from build123d import *

# Parameters (mm, degrees)
BOSS_EXTRUDE1_DEPTH     = 202
FILLET1_R               = 1.44
FILLET2_R               = 1.44
SKETCH2_R               = 1.59
SKETCH2_R_2             = 1.735
SKETCH2_R_3             = 1.57
CUT_EXTRUDE1_DEPTH      = 6.1
CUT_EXTRUDE1_DEPTH_BACK = 11.04
FILLET3_R               = 1.44
BOSS_EXTRUDE2_DEPTH     = 202
CUT_EXTRUDE2_DEPTH      = 203
SKETCH5_R               = 1.59
CUT_EXTRUDE3_DEPTH      = 10
SKETCH6_R               = 1.59
BOSS_EXTRUDE3_DEPTH     = 1.59


with BuildPart() as part:
    # Sketch1 → Boss-Extrude1 (new body)
    with BuildSketch(Plane(origin=(0, 0, 0), x_dir=(0, 0, -1), z_dir=(1, 0, 0))):
        with BuildLine():
            Line((-15.04, 0), (15.04, 0))
            Line((15.04, 0), (15.19, 0))
            ThreePointArc((15.19, 0), (16.208233765, 0.421766235), (16.63, 1.44))
            Line((16.63, 1.44), (16.63, 12.11))
            ThreePointArc((16.63, 12.11), (17.051766235, 13.128233765), (18.07, 13.55))
            Line((18.07, 13.55), (24.5, 13.55))
            Line((24.5, 13.55), (24.5, 15.14))
            Line((24.5, 15.14), (16.48, 15.14))
            ThreePointArc((16.48, 15.14), (15.461766235, 14.718233765), (15.04, 13.7))
            Line((15.04, 13.7), (15.04, 3.03))
            ThreePointArc((15.04, 3.03), (14.618233765, 2.011766235), (13.6, 1.59))
            Line((13.6, 1.59), (-13.6, 1.59))
            ThreePointArc((-13.6, 1.59), (-14.618233765, 2.011766235), (-15.04, 3.03))
            Line((-15.04, 3.03), (-15.04, 8.6))
            ThreePointArc((-15.04, 8.6), (-15.461766235, 9.618233765), (-16.48, 10.04))
            Line((-16.48, 10.04), (-24.68, 10.04))
            Line((-24.68, 10.04), (-24.68, 8.45))
            Line((-24.68, 8.45), (-18.07, 8.45))
            ThreePointArc((-18.07, 8.45), (-17.051766235, 8.028233765), (-16.63, 7.01))
            Line((-16.63, 7.01), (-16.63, 1.44))
            ThreePointArc((-16.63, 1.44), (-16.208233765, 0.421766235), (-15.19, 0))
            Line((-15.19, 0), (-15.04, 0))
        make_face()
    extrude(amount=-BOSS_EXTRUDE1_DEPTH)

    # Fillet1
    fillet1_edges = [part.edges().sort_by_distance(p)[0] for p in [
        (0, 9.245, 24.68),
    ]]
    fillet(fillet1_edges, radius=FILLET1_R)

    # Fillet2
    fillet2_edges = [part.edges().sort_by_distance(p)[0] for p in [
        (-202, 14.345, -24.5),
        (0, 14.345, -24.5),
        (-202, 9.245, 24.68),
    ]]
    fillet(fillet2_edges, radius=FILLET2_R)

    # Sketch2 → Cut-Extrude1 (cut, two sides)
    with BuildSketch(Plane(origin=(0, 10.04, 0), x_dir=(1, 0, 0), z_dir=(0, 1, 0))) as cut_extrude1_sk:
        with Locations((-193.95, -20.6)):
            Circle(SKETCH2_R)
        with Locations((-8.05, -20.6)):
            Circle(SKETCH2_R)
        with Locations((-176.235, 1.415)):
            Circle(SKETCH2_R_2)
        with Locations((-25.765, 1.415)):
            Circle(SKETCH2_R_2)
        with Locations((-193.91, 20.563)):
            Circle(SKETCH2_R)
        with Locations((-101, 1.31)):
            Circle(SKETCH2_R_3)
        with Locations((-8.09, 20.563)):
            Circle(SKETCH2_R)
        with BuildLine():
            Line((0, 4.455), (0, -4.455))
            Line((0, -4.455), (-3.9, -4.455))
            ThreePointArc((-3.9, -4.455), (-8.355, 0), (-3.9, 4.455))
            Line((-3.9, 4.455), (0, 4.455))
        make_face()
        with BuildLine():
            Line((-141.669852281, -24.68), (-141.669852281, -22.87))
            ThreePointArc((-141.669852281, -22.87), (-139.919852281, -21.12), (-138.169852281, -22.87))
            Line((-138.169852281, -22.87), (-138.169852281, -24.68))
            Line((-138.169852281, -24.68), (-141.669852281, -24.68))
        make_face()
        with BuildLine():
            Line((-63.830147719, -22.87), (-63.830147719, -24.68))
            Line((-63.830147719, -24.68), (-60.330147719, -24.68))
            Line((-60.330147719, -24.68), (-60.330147719, -22.87))
            ThreePointArc((-60.330147719, -22.87), (-62.080147719, -21.12), (-63.830147719, -22.87))
        make_face()
        with BuildLine():
            Line((-139.73, 24.5), (-136.23, 24.5))
            Line((-136.23, 24.5), (-136.23, 22.6))
            ThreePointArc((-136.23, 22.6), (-137.98, 20.85), (-139.73, 22.6))
            Line((-139.73, 22.6), (-139.73, 24.5))
        make_face()
        with BuildLine():
            Line((-202, 4.455), (-202, -4.455))
            Line((-202, -4.455), (-198.1, -4.455))
            ThreePointArc((-198.1, -4.455), (-193.645, 0), (-198.1, 4.455))
            Line((-198.1, 4.455), (-202, 4.455))
        make_face()
        with BuildLine():
            Line((-62.27, 24.5), (-62.27, 22.6))
            ThreePointArc((-62.27, 22.6), (-64.02, 20.85), (-65.77, 22.6))
            Line((-65.77, 22.6), (-65.77, 24.5))
            Line((-65.77, 24.5), (-62.27, 24.5))
        make_face()
    extrude(amount=CUT_EXTRUDE1_DEPTH, mode=Mode.SUBTRACT)
    extrude(cut_extrude1_sk.sketch, amount=-CUT_EXTRUDE1_DEPTH_BACK, mode=Mode.SUBTRACT)

    # Fillet3
    fillet3_edges = [part.edges().sort_by_distance(p)[0] for p in [
        (-202, 0.795, 4.455),
        (-202, 0.795, -4.455),
        (0, 0.795, -4.455),
        (0, 0.795, 4.455),
    ]]
    fillet(fillet3_edges, radius=FILLET3_R)

    # Sketch3 → Boss-Extrude2 (add)
    with BuildSketch(Plane.ZY.offset(202)):
        with BuildLine():
            Line((15.04, 3.03), (15.04, 8.6))
            ThreePointArc((15.04, 8.6), (15.461766235, 9.618233765), (16.48, 10.04))
            Line((16.48, 10.04), (12.551925622, 10.038202595))
            ThreePointArc((12.551925622, 10.038202595), (11.487521511, 9.643353463), (11.04, 8.6))
            Line((11.04, 8.6), (11.04, 3.03))
            ThreePointArc((11.04, 3.03), (10.618233765, 2.011766235), (9.6, 1.59))
            Line((9.6, 1.59), (13.6, 1.59))
            ThreePointArc((13.6, 1.59), (14.618233765, 2.011766235), (15.04, 3.03))
        make_face()
    extrude(amount=-BOSS_EXTRUDE2_DEPTH)

    # Sketch4 → Cut-Extrude2 (cut, through all)
    with BuildSketch(Plane.ZY.offset(202)):
        with BuildLine():
            Line((16.63, 7.01), (16.63, 1.44))
            ThreePointArc((16.63, 1.44), (16.208233765, 0.421766235), (15.19, 0))
            Line((15.19, 0), (11.19, 0))
            ThreePointArc((11.19, 0), (12.208233765, 0.421766235), (12.63, 1.44))
            Line((12.63, 1.44), (12.63, 7.01))
            ThreePointArc((12.63, 7.01), (13.051766235, 8.028233765), (14.07, 8.45))
            Line((14.07, 8.45), (18.07, 8.45))
            ThreePointArc((18.07, 8.45), (17.051766235, 8.028233765), (16.63, 7.01))
        make_face()
    extrude(amount=-CUT_EXTRUDE2_DEPTH, mode=Mode.SUBTRACT)

    # Sketch5 → Cut-Extrude3 (cut)
    with BuildSketch(Plane(origin=(0, 10.04, 0), x_dir=(1, 0, 0), z_dir=(0, 1, 0))):
        with Locations((-193.95, -20.6)):
            Circle(SKETCH5_R)
        with Locations((-8.05, -20.6)):
            Circle(SKETCH5_R)
        with Locations((-193.95, -16.6)):
            Circle(SKETCH5_R)
        with Locations((-8.05, -16.6)):
            Circle(SKETCH5_R)
    extrude(amount=-CUT_EXTRUDE3_DEPTH, mode=Mode.SUBTRACT)

    # Sketch6 → Boss-Extrude3 (add)
    with BuildSketch(Plane(origin=(0, 10.04, 0), x_dir=(1, 0, 0), z_dir=(0, 1, 0))):
        with Locations((-193.95, -20.6)):
            Circle(SKETCH6_R)
        with Locations((-8.05, -20.6)):
            Circle(SKETCH6_R)
    extrude(amount=-BOSS_EXTRUDE3_DEPTH)


solid = part.part
For this review, take the finished solid that the model builds, in its own axes (mm). A direction names the side the tool comes from. Round coordinates to 2 decimals unless told otherwise and drop trailing zeros. Write each loop counter-clockwise with the first axis right and the second up, starting at its lowest first coordinate (ties: lowest second). Pieces come first, ordered by that corner, then holes. Notation, with made-up numbers: (29, -26) -> (88, -26) arc R30 ccw to (88, 9) -> close; hole circle Ø6 at (48.25, -14.5). An arc over 180 degrees is marked (long way). Put each result on its own line as item: value.
Q1. Consider section A-A on x = -57.5. State the section outline as (y, z) points.
Determined:
outline: (0, -15.19) arc R1.44 ccw to (1.44, -16.63) -> (12.11, -16.63) arc R1.44 cw to (13.55, -18.07) -> (13.55, -24.5) -> (15.14, -24.5) -> (15.14, -16.48) arc R1.44 ccw to (13.7, -15.04) -> (3.03, -15.04) arc R1.44 cw to (1.59, -13.6) -> (1.59, 9.6) arc R1.44 cw to (3.03, 11.04) -> (8.6, 11.04) arc R1.44 ccw to (10.04, 12.55) -> (10.04, 16.48) -> (10.04, 24.68) -> (8.45, 24.68) -> (8.45, 14.07) arc R1.44 cw to (7.01, 12.63) -> (1.44, 12.63) arc R1.44 ccw to (0, 11.19) -> close
Q2. Consider section B-B on z = -11. State the section outline as (x, y) points, and give its area (3 significant figures).
Determined:
outline: (-202, 0) -> (0, 0) -> (0, 1.59) -> (-202, 1.59) -> close
area: 321 mm^2
Q3. To check wall thickness, follow L1, parallel to Z at x = -83, y = 6.5; L2, parallel to Z at x = -8.05, y = 8.85; L3, parallel to X at y = 1.2, z = -1.31. State the ranges of each line that lie inside material, in increasing order. Write a range as [from, to].
Determined:
L1: z = [-16.63, -15.04], [11.04, 12.63]
L2: z = [-16.63, -15.04], [11.06, 15.01], [18.19, 24.68]
L3: x = [-193.84, -177.97], [-174.5, -102.57], [-99.43, -27.5], [-24.03, -8.16]
Q4. The part is to be moulded in two halves that separate along Z. For faces 1 (the flat face through (-100, 7, -16.63)), 2 (the flat face through (0, 6, 12)), 3 (the cylindrical face through (-8.354, 0.806, 0.098)), say which applies: released by +Z, released by -Z, zero draft, split by the parting line, or undercut.
Determined:
face 1: released by -Z
face 2: zero draft
face 3: undercut
Q5. Machinability: for faces 4 (the flat face through (-102, 6, 11.04)), 5 (the flat face through (-100, 8.45, 19)), 6 (the flat face through (-100, 13.55, -21)), which of the approach directions +Z, -Z, +X, -X, +Y, -Y give a long, thin tool a straight path to every point of the face, cutting with its end or side? Answer none if there is none.
Determined:
face 4: +X, -X, +Y
face 5: +Z, +X, -X, -Y
face 6: -Z, +X, -X, -Y
Q6. Clearance check with flat-ended pins moving along their axes: pin 1 Ø5 at (x, y) = (-107.5, 9) entering from -Z; pin 2 Ø3 at (x, z) = (-25.765, -1.415) entering from +Y; pin 3 Ø0.5 at (x, y) = (-2.5, 0.5) entering from -Z; pin 4 Ø1 at (x, z) = (-123, -15) entering from +Y. State where each tip first meets the part, or that it passes through.
Determined:
pin 1: stops at z = -16.63
pin 2: passes through
pin 3: stops at z = -16.45
pin 4: stops at y = 14.76
